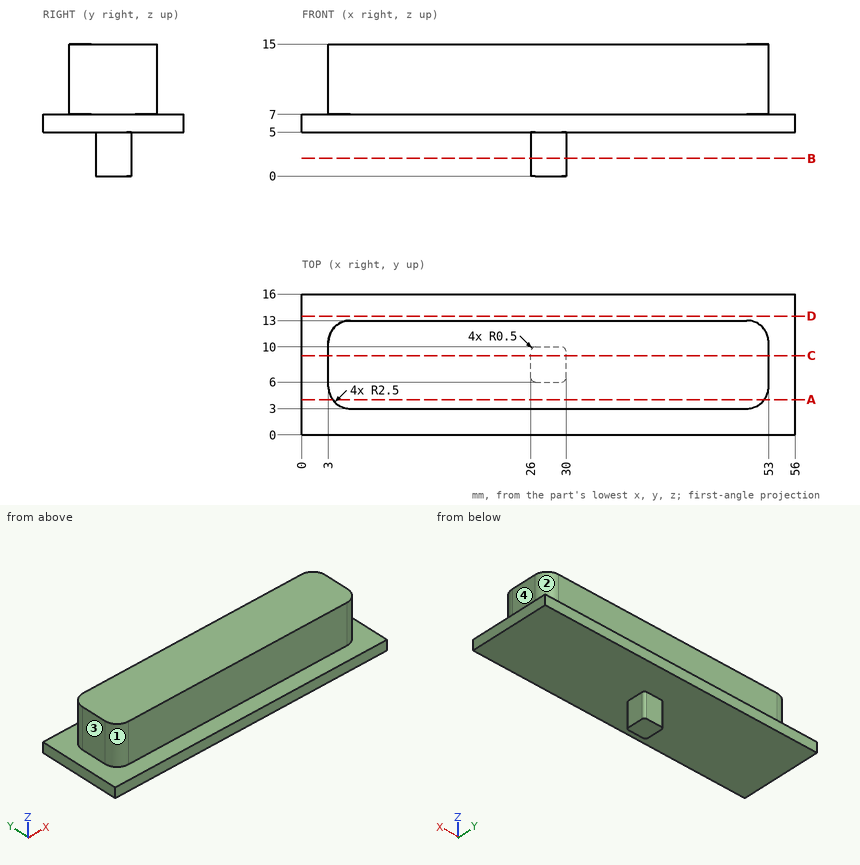
Check sheet for the drawn part. Datum: minimum x, y, z corner. Units: mm. A direction names the side the tool comes from. Round coordinates to 2 decimals unless told otherwise and drop trailing zeros. Order: outer loops, then holes, each group sorted by start corner. A loop starts at its lowest first (then second) coordinate and runs counter-clockwise, first axis right, second up.
(1) Cross-section at A-A, the plane y = 4. Enter the section's corners in (x, z).
(2) Go/stop test with flat-tipped pins: P1, Ø2.5, axis at y = 7.5, z = 2.5, coming from the -X side; P2, Ø2.5, axis at x = 27.5, z = 1.5, coming from the +Y side; P3, Ø2.5, axis at x = 17.5, z = 12.5, coming from the -Y side. Record where each tip stops, or that it passes through.
(3) Scan lines: probe 1 along Z at (x, y) = (18, 6); probe 2 along Z at (x, y) = (48, 13.5); probe 3 along Y at (x, z) = (17.5, 12.75). Record each from-to range of solid material in increasing order.
(4) Cross-section at D-D, the plane y = 13.5. Enter the section's corners in (x, z), and give its area (3 significant figures).
(5) Access from +Z, -Z, +X, -X, +Y, -Y to the whole of each face (thin tool, end or side, straight path). Record for the marked faces 1, 2, 3 and 4.
(6) Cross-section at B-B, the plane z = 2. Enter the section's corners in (x, y).
(7) Cross-section at C-C, the plane y = 9. Enter the section's corners in (x, z).
Check sheet entries:
1. outline: (0, 5) - (56, 5) - (56, 7) - (52.5, 7) - (52.5, 15) - (3.5, 15) - (3.5, 7) - (0, 7) - close
2. P1: stops at x = 26
2. P2: stops at y = 10
2. P3: stops at y = 3
3. probe 1: z = 5 to 15
3. probe 2: z = 5 to 7
3. probe 3: y = 3 to 13
4. outline: (0, 5) - (56, 5) - (56, 7) - (0, 7) - close
4. area: 112 mm2
5. face 1: +Z, -X, -Y
5. face 2: +Z, +X, +Y
5. face 3: +Z, -X, +Y, -Y
5. face 4: +Z, +X, +Y, -Y
6. outline: (26, 6.5) arc R0.5 ccw to (26.5, 6) - (29.5, 6) arc R0.5 ccw to (30, 6.5) - (30, 9.5) arc R0.5 ccw to (29.5, 10) - (26.5, 10) arc R0.5 ccw to (26, 9.5) - close
7. outline: (0, 5) - (26, 5) - (26, 0) - (30, 0) - (30, 5) - (56, 5) - (56, 7) - (53, 7) - (53, 15) - (3, 15) - (3, 7) - (0, 7) - close
